Geometry: final body of the model. Coordinates: model frame, mm. Face numbers are marked on the shaded views. Give positions to 0.01 mm unless a question says otherwise; leave off trailing zeros. Loops run counter-clockwise (first coordinate to the right, second up) from the corner with the lowest first, then second, coordinate; pieces in that order, holes last.
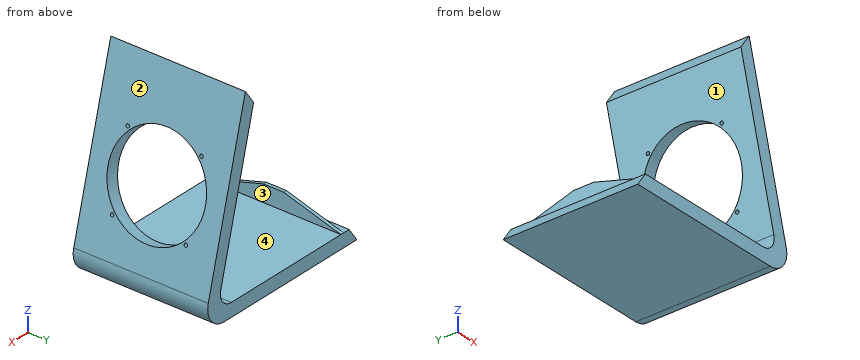
```python
from build123d import *

# Parameters (mm, degrees)
F1_DEPTH = 200
F2_R     = 72.5
F2_R_2   = 2.5
F3_DEPTH = 20
F4_R     = 20
F5_R     = 30
F6_W     = 5
F6_H     = 200
F7_DEPTH = 25
F9_DEPTH = 25


with BuildPart() as f1:
    # F0 (on Front) → F1 (new body)
    with BuildSketch(Plane.XZ):
        Polygon((14.0041507642, 20), (0, 0), (280.5502770065, 0), (202.9045634757, 289.7777478867), (187.9295462557, 268.391206893), (254.4857695496, 20), align=None)
    extrude(amount=F1_DEPTH)

    # F2 (on face) → F3 (cut, through all)
    with BuildSketch(Plane(origin=(261.7569719664, 0, 70.1375692516), x_dir=(0, 1, 0), z_dir=(0.9659258263, 0, 0.2588190451))):
        with Locations((-100, 77.3882452019)):
            Circle(F2_R)
        with Locations((-154.8, 132.1882452019)):
            Circle(F2_R_2)
        with Locations((-45.2, 132.1882452019)):
            Circle(F2_R_2)
        with Locations((-45.2, 22.5882452019)):
            Circle(F2_R_2)
        with Locations((-154.8, 22.5882452019)):
            Circle(F2_R_2)
    extrude(amount=-F3_DEPTH, mode=Mode.SUBTRACT)

    # F4
    f4_edges = [f1.edges().sort_by_distance(p)[0] for p in [
        (254.48577, -100, 20),
    ]]
    fillet(f4_edges, radius=F4_R)

    # F5
    f5_edges = [f1.edges().sort_by_distance(p)[0] for p in [
        (280.550277, -100, 0),
    ]]
    fillet(f5_edges, radius=F5_R)

    # F6 (on face) → F7 (join)
    with BuildSketch(Plane.XY.offset(20)):
        with Locations((26.5041507642, -100)):
            Rectangle(F6_W, F6_H)
    extrude(amount=F7_DEPTH)

    # F8 (on face) → F9 (cut)
    with BuildSketch(Plane(origin=(24.0041507642, 0, 0), x_dir=(0, -1, 0), z_dir=(-1, 0, 0))):
        Polygon((0, 20), (85, 45), (0, 45), align=None)
        Polygon((200, 45), (115, 45), (200, 20), align=None)
    extrude(amount=-F9_DEPTH, mode=Mode.SUBTRACT)


solid = f1.part
```
Q1. Section query A-A, the plane y = -60.5. Return loops of the section in (x, z), and give its area (3 significant figures).
Q2. Material intervals for probe 1 along Z at (x, y) = (78.5, -171); probe 2 along X at (y, z) = (-47.5, 28.5); probe 3 along X at (y, z) = (-104, 68.5), sorted ascending.
Q3. Mould query, pull axis Z, two halves, no side actions, for the marked faces 1, 2, 3 and 4. Classes: +Z half, -Z half, draft (parallel to the pull), parting line (faces both ways), or undercut.
Q4. Section query B-B, the plane x = 93. Return loops of the section in (y, z), and give its area (3 significant figures).
Q5. Section query D-D, the plane y = -133. Return loops of the section in (x, z), and give its area (3 significant figures).
Q6. Pin query (flat end, axial travel): pin 1 Ø6 at (y, z) = (-178.5, 119.5) entering from -X; pin 2 Ø4 at (x, y) = (27, -93.5) entering from +Z. Return the tip coordinate at first contact, or that it passes through.
Q7. Section query C-C, the plane y = -185. Return loops of the section in (x, z).
Resolved:
1. outline: (0, 0) - (241.45, 0) arc R30 ccw to (270.43, 37.76) - (257.46, 86.17) - (238.14, 80.99) - (247.74, 45.18) arc R20 cw to (228.42, 20) - (29, 20) - (29, 37.79) - (24, 37.79) - (24, 20) - (14, 20) - close; (187.93, 268.39) - (206.67, 198.44) - (225.99, 203.61) - (202.9, 289.78) - close
1. area: 8,250 mm2
2. probe 1: z = 0 to 20
2. probe 2: x = 24 to 29, 244.78 to 271.42
2. probe 3: x = 241.49 to 262.2
3. face 1: undercut
3. face 2: +Z half
3. face 3: draft
3. face 4: undercut
4. outline: (-200, 0) - (0, 0) - (0, 20) - (-200, 20) - close
4. area: 4,000 mm2
5. outline: (0, 0) - (241.45, 0) arc R30 ccw to (270.43, 37.76) - (258.44, 82.53) - (239.12, 77.36) - (247.74, 45.18) arc R20 cw to (228.42, 20) - (29, 20) - (29, 39.71) - (24, 39.71) - (24, 20) - (14, 20) - close; (187.93, 268.39) - (205.7, 202.07) - (225.02, 207.24) - (202.9, 289.78) - close
5. area: 8,100 mm2
6. pin 1: stops at x = 227.02
6. pin 2: stops at z = 45
7. outline: (0, 0) - (241.45, 0) arc R30 ccw to (270.43, 37.76) - (202.9, 289.78) - (187.93, 268.39) - (247.74, 45.18) arc R20 cw to (228.42, 20) - (29, 20) - (29, 24.41) - (24, 24.41) - (24, 20) - (14, 20) - close
